from build123d import *

# Parameters (mm, degrees)
SKIZZE1_R                       = 2.5
AUFSATZ_LINEAR_AUSTRAGEN1_DEPTH = 6
SKIZZE2_W                       = 5.35
SKIZZE2_H                       = 26.25
SCHNITT_LINEAR_AUSTRAGEN1_DEPTH = 3
SKIZZE3_W                       = 55
SKIZZE3_H                       = 20
SCHNITT_LINEAR_AUSTRAGEN2_DEPTH = 2
VERRUNDUNG1_R                   = 3
FASE1_SIZE                      = 2


with BuildPart() as part:
    # Skizze1 → Aufsatz-Linear austragen1 (new body)
    with BuildSketch(Plane(origin=(0, 0, 0), x_dir=(1, 0, 0), z_dir=(0, 1, 0))):
        Polygon((-27.5, -75), (-27.5, 75), (-7, 75), (-7, 89), (7, 89), (7, 75), (27.5, 75), (27.5, -75), (7, -75), (7, -89), (-7, -89), (-7, -75), align=None)
        with Locations(Location((0, 82, 0), (0, 0, 270))):
            Circle(SKIZZE1_R, mode=Mode.SUBTRACT)
        with Locations(Location((0, -82, 0), (0, 0, 90))):
            Circle(SKIZZE1_R, mode=Mode.SUBTRACT)
    extrude(amount=AUFSATZ_LINEAR_AUSTRAGEN1_DEPTH)

    # Skizze2 → Schnitt-Linear austragen1 (cut)
    with BuildSketch(Plane(origin=(0, 6, 0), x_dir=(1, 0, 0), z_dir=(0, 1, 0))):
        with Locations((-21.575, 20.125)):
            Rectangle(SKIZZE2_W, SKIZZE2_H)
        with Locations((21.575, 20.125)):
            Rectangle(SKIZZE2_W, SKIZZE2_H)
        with Locations((-21.575, -43.125)):
            Rectangle(SKIZZE2_W, SKIZZE2_H)
        with Locations((21.575, -43.125)):
            Rectangle(SKIZZE2_W, SKIZZE2_H)
    extrude(amount=-SCHNITT_LINEAR_AUSTRAGEN1_DEPTH, mode=Mode.SUBTRACT)

    # Skizze3 → Schnitt-Linear austragen2 (cut)
    with BuildSketch(Plane.XZ):
        with Locations((0, 12)):
            Rectangle(SKIZZE3_W, SKIZZE3_H)
    extrude(amount=-SCHNITT_LINEAR_AUSTRAGEN2_DEPTH, mode=Mode.SUBTRACT)

    # Verrundung1
    verrundung1_edges = [part.edges().sort_by_distance(p)[0] for p in [
        (-7, 3, -75),
        (-7, 3, -89),
        (7, 3, -89),
        (7, 3, -75),
        (27.5, 3, -75),
        (27.5, 3, 75),
        (7, 3, 75),
        (7, 3, 89),
        (-7, 3, 89),
        (-7, 3, 75),
        (-27.5, 3, 75),
        (-27.5, 3, -75),
    ]]
    fillet(verrundung1_edges, radius=VERRUNDUNG1_R)

    # Fase1
    fase1_edges = [part.edges().sort_by_distance(p)[0] for p in [
        (0, 0, 22),
        (0, 0, 2),
    ]]
    chamfer(fase1_edges, length=FASE1_SIZE - 0.0001)  # a hair under: the kernel refuses the full size


solid = part.part
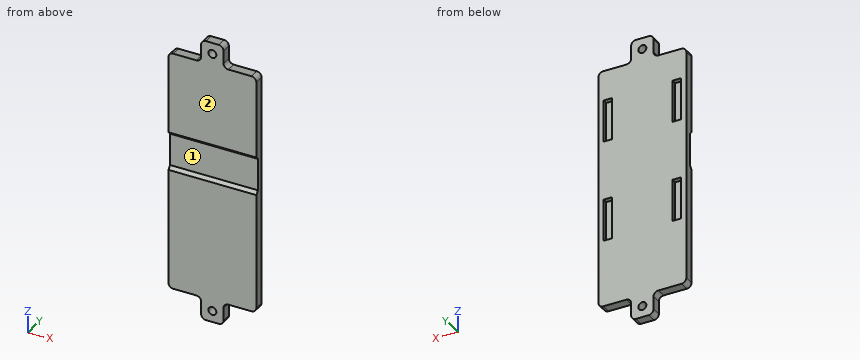
Design review of the part built by this model. Coordinates are the model's own, in mm. Face numbers are marked on the shaded views. Coordinates: 2 decimals unless noted, no trailing zeros. Order: outer loops, then holes, each group sorted by start corner. A loop starts at its lowest first (then second) coordinate and runs counter-clockwise, first axis right, second up. Notation, with made-up numbers: (13, -30.5) -> (38, -30.5) arc R13 cw to (38, -25.5) -> close; hole circle Ø7 at (-11, 50.25). An arc over 180 degrees is marked (long way). Use one line per item in the form item = value. Start each with the question number.
(1) Insertion check: pin 1 (3.5 mm diameter, centred on x = -21.5, y = 4.5, fed in from +Z); pin 2 (6 mm diameter, centred on x = 0, z = 82, fed in from +Y); pin 3 (3 mm diameter, centred on x = 15, y = 3, fed in from -Z); pin 4 (1.6 mm diameter, centred on x = 20.5, z = -26, fed in from +Y). Each pin has a flat end and moves straight along its axis. Give the tip position at first contact, or say it passes through.
(2) The part is to be moulded in two halves that separate along Z. For the marked faces 1 and 2, say which applies: +Z half, -Z half, draft (parallel to the pull), parting line (faces both ways), or undercut.
(3) For probe 1 along Z at (x, y) = (19, 4.1); probe 2 along X at (y, z) = (4.75, -23); probe 3 along X at (y, z) = (3.35, -82), list the stretches that pass through material, from the lowest coordinate up.
(4) Add section A-A on z = 82. State the section outline as (x, y) points, plus the area to 3 significant figures.
(5) Add section B-B on x = 0. Give the number of separate pieces and of enclosed holes in the cut face, plus the area to 3 significant figures.
Answer block:
q1.pin_1 = 75
q1.pin_2 = 6
q1.pin_3 = -75
q1.pin_4 = 3
q2.face_1 = undercut
q2.face_2 = draft
q3.probe_1 = -75 to -33.25, -7 to 30, 56.25 to 75
q3.probe_2 = -27.5 to -24.25, -18.9 to 18.9, 24.25 to 27.5
q3.probe_3 = -7 to -2.5, 2.5 to 7
q4.outline = (-7, 0) -> (-2.5, 0) -> (-2.5, 6) -> (-7, 6) -> close; (2.5, 0) -> (7, 0) -> (7, 6) -> (2.5, 6) -> close
q4.area = 54.0 mm²
q5.separate_pieces = 3
q5.enclosed_holes = 0
q5.area = 964 mm²
